For this review, use the dimensioned drawing (mm, ordinates from the lowest corner) and the shaded views. A direction names the side the tool comes from. Coordinates: 2 decimals unless noted, no trailing zeros. Loops run counter-clockwise (first coordinate to the right, second up) from the corner with the lowest first, then second, coordinate; pieces in that order, holes last. Notation, with made-up numbers: M -30.75,51.25 L 17.25,51.25 A27 ccw 17.25,74.25 Z; hole C 67,30 d11. An arc over 180 degrees is marked long. Use CSV: the item, a comma, the result in double quotes. Start each with the question number.
1. Draft analysis for pull direction X (two halves, no side actions). For the marked faces 4, 5 and 6, state which applies: +X half, -X half, draft (parallel to the pull), parting line (faces both ways), or undercut.
2. For L1, parallel to X at y = 25, z = 48; L2, parallel to Y at x = 32, z = 66; L3, parallel to Y at x = 67, z = 22, list the stretches that pass through material, from the lowest coordinate up.
3. Add section B-B, the plane y = 46. Write out the cut boundary in (x, z).
4. Add section C-C, the plane z = 47.5. Write out the cut boundary in (x, y), then the cut area to 3 significant figures.
5. Tool access review of the marked faces 1, 2 and 3: name each direction out of +Z, -Z, +X, -X, +Y, -Y from which nothing blocks a thin tool from reaching the whole face with its end or side.
6. Clearance check with flat-ended pins moving along their axes: P1, Ø2.5, axis at y = 34.5, z = 75.5, coming from the +X side; P2, Ø15, axis at x = 28, y = 63, coming from the +Z side; P3, Ø9, axis at y = 54, z = 89, coming from the -X side. State where each tip first meets the part, or that it passes through.
7. Add section A-A, the plane x = 36. Write out the cut boundary in (y, z), then the cut area to 3 significant figures.
8. Add section D-D, the plane z = 75.5. Write out the cut boundary in (x, y), then the cut area to 3 significant figures.
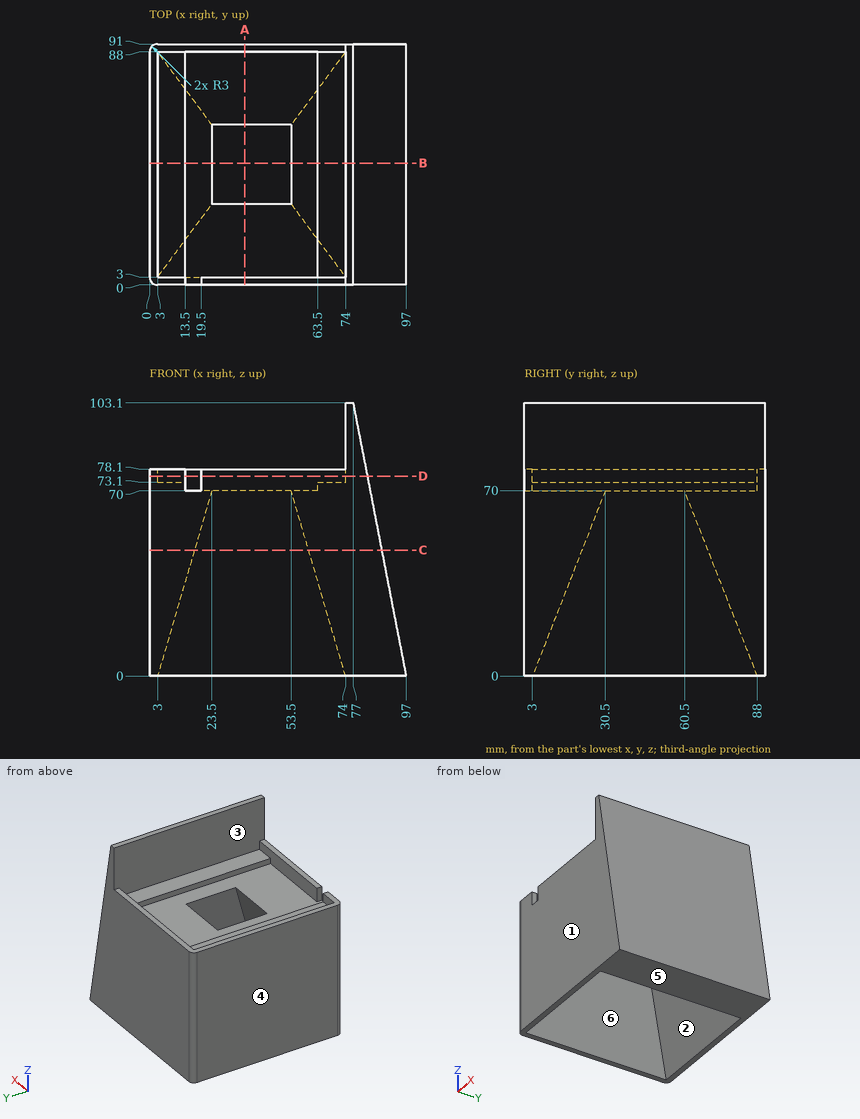
Computed:
1,face 4,"-X half"
1,face 5,"draft"
1,face 6,"undercut"
2,L1,"x = 0 to 17.06, 59.94 to 87.69"
2,L2,"y = 0 to 28.93, 62.07 to 91"
2,L3,"y = 0 to 11.64, 79.36 to 91"
3,outline,"M 0,0 L 3,0 L 23.5,70 L 13.5,70 L 13.5,73.1 L 3,73.1 L 3,78.1 L 0,78.1 Z; M 53.5,70 L 74,0 L 97,0 L 77,103.1 L 74,103.1 L 74,73.1 L 63.5,73.1 L 63.5,70 Z"
4,outline,"M 0,3 A3 ccw 3,0 L 87.79,0 L 87.79,91 L 3,91 A3 ccw 0,88 Z; hole M 16.91,21.66 L 60.09,21.66 L 60.09,69.34 L 16.91,69.34 Z"
4,area,"5,930 mm^2"
5,face 1,"+Z, -Z, +X, -X, -Y"
5,face 2,"-Z"
5,face 3,"+Z"
6,P1,"stops at x = 82.6"
6,P2,"stops at z = 70"
6,P3,"stops at x = 74"
7,outline,"M 0,0 L 3,0 L 30.5,70 L 3,70 L 3,78.1 L 0,78.1 Z; M 60.5,70 L 88,0 L 91,0 L 91,78.1 L 88,78.1 L 88,70 Z"
7,area,"2,390 mm^2"
8,outline,"M 0,3 A3 ccw 3,0 L 13.5,0 L 13.5,3 L 3,3 L 3,88 L 74,88 L 74,3 L 19.5,3 L 19.5,0 L 82.35,0 L 82.35,91 L 3,91 A3 ccw 0,88 Z"
8,area,"1,440 mm^2"
